Check sheet for the modelled part. Datum: model origin and axes. Units: mm. Round coordinates to 2 decimals unless told otherwise and drop trailing zeros. Write each loop counter-clockwise with the first axis right and the second up, starting at its lowest first coordinate (ties: lowest second). Pieces come first, ordered by that corner, then holes. Notation, with made-up numbers: (29.5, 36.25) -> (52.5, 36.25) arc R30 cw to (52.5, 64.25) -> close; hole circle Ø4 at (70, 49). An arc over 180 degrees is marked (long way). Write item = value, one per line.
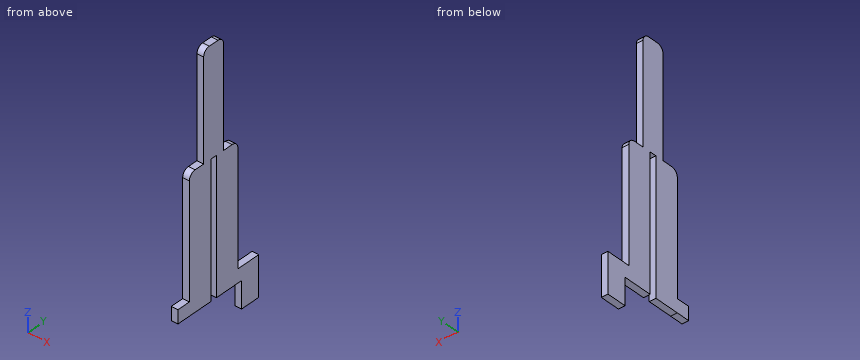
from build123d import *

# Parameters (mm, degrees)
F1_DEPTH = 3.175


with BuildPart() as f1:
    # F0 (on Right) → F1 (new body, symmetric)
    with BuildSketch(Plane.YZ):
        with BuildLine():
            Line((3.175, -63.5), (26.9875, -63.5))
            Line((26.9875, -63.5), (26.9875, -50.8))
            Line((26.9875, -50.8), (26.9875, 57.15))
            ThreePointArc((26.9875, 57.15), (25.127628, 61.640128), (20.6375, 63.5))
            Line((20.6375, 63.5), (17.464617, 63.5))
            Line((17.464617, 63.5), (11.113911, 63.5))
            Line((11.113911, 63.5), (11.124494, 158.749293))
            ThreePointArc((11.124494, 158.749293), (9.264872, 163.239877), (4.774494, 165.099999))
            Line((4.774494, 165.099999), (-4.7498, 165.099999))
            ThreePointArc((-4.7498, 165.099999), (-9.239928, 163.240127), (-11.0998, 158.749999))
            Line((-11.0998, 158.749999), (-11.0998, 63.5))
            Line((-11.0998, 63.5), (-17.4498, 63.5))
            Line((-17.4498, 63.5), (-20.6375, 63.5))
            ThreePointArc((-20.6375, 63.5), (-25.127628, 61.640128), (-26.9875, 57.15))
            Line((-26.9875, 57.15), (-26.9875, -50.818807))
            Line((-26.9875, -50.818807), (-26.9875, -63.5))
            Line((-26.9875, -63.5), (-3.175, -63.5))
            Line((-3.175, -63.5), (-3.175, 63.5))
            Line((-3.175, 63.5), (3.175, 63.5))
            Line((3.175, 63.5), (3.175, -63.5))
        make_face()
        Polygon((26.9875, -50.8), (26.9875, -63.5), (31.115, -63.5), (31.115, -88.9), (50.165, -88.9), (50.165, -50.8), align=None)
        Polygon((-39.6875, -63.518807), (-26.9875, -63.5), (-26.9875, -50.818807), (-39.6875, -50.818807), align=None)
    extrude(amount=F1_DEPTH, both=True)


solid = f1.part
(1) Sectioned sample at D-D on z = 120.5. Enter the section's corners in (x, y) (3 decimals).
Worked answers:
outline = (-3.175, -11.1) -> (3.175, -11.1) -> (3.175, 11.12) -> (-3.175, 11.12) -> close
(2) Sectioned sample at C-C on y = 14. Enter the section's corners in (x, z) (3 decimals).
Worked answers:
outline = (-3.175, -63.5) -> (3.175, -63.5) -> (3.175, 63.5) -> (-3.175, 63.5) -> close
(3) Sectioned sample at A-A on z = 37. Enter the section's corners in (x, y) (1 decimal).
Worked answers:
outline = (-3.2, -27) -> (3.2, -27) -> (3.2, -3.2) -> (-3.2, -3.2) -> close; (-3.2, 3.2) -> (3.2, 3.2) -> (3.2, 27) -> (-3.2, 27) -> close
(4) Material ranges on L1, parallel to Y at x = -1, z = 51.5 (1 decimal); L2, parallel to Z at x = 0.25, y = -4.5; L3, parallel to Z at x = -2.25, y = -18, recorded low to high. Write a range as [from, to].
Worked answers:
L1 = [-27, -3.2], [3.2, 27]
L2 = [-63.5, 165.1]
L3 = [-63.5, 63.5]
(5) Go/stop test with flat-tipped pins: P1, Ø1.9, axis at x = -0.5, y = 0.5, coming from the -Z side; P2, Ø1.9, axis at x = -0.5, z = 123.5, coming from the +Y side; P3, Ø1.5, axis at x = 2, z = 0.5, coming from the -Y side. Record where each tip stops, or that it passes through.
Worked answers:
P1 = 63.5
P2 = 11.12
P3 = -26.99
